Build history of the part. All positions in model axes, mm. A direction names the side the tool comes from. Round coordinates to 2 decimals unless told otherwise and drop trailing zeros. Write each loop counter-clockwise with the first axis right and the second up, starting at its lowest first coordinate (ties: lowest second). Pieces come first, ordered by that corner, then holes.
1) Which spindle directions (+Z, -Z, +X, -X, +Y, -Y) get a long thin tool onto all of the face, cutting with end or side? Do faces 4 (the flat face through (15.76, -5.42, -0.91)), 5 (the flat face through (14, -11, -12)), 6 (the flat face through (16.257, -5.423, -9.902)). Say none if no direction does.
2) Flat gauge pins, fed straight in: pin 1 (4 mm diameter, centred on y = -5.5, z = -5, fed in from -X); pin 2 (6 mm diameter, centred on x = 1.5, y = -4, fed in from -Z); pin 3 (1 mm diameter, centred on y = -2, z = -7, fed in from +X); pin 4 (14 mm diameter, centred on x = -4.5, z = -2, fed in from -Y). Where does each tip first touch, or does it go through?
3) Saw through at D-D (x = 19.5). Write the cut outline in (y, z).
4) Wall check: probe 1 along Y at (x, z) = (9, 7.75); probe 2 along X at (y, z) = (0.35, 0); probe 3 along Z at (x, y) = (14, -1). Give the ranges that are in metal, low to high.
5) Saw through at A-A (y = -7). Write the cut outline in (x, z).
6) Saw through at C-C (z = -8). Write the cut outline in (x, y).
7) Saw through at B-B (x = -6). Write the cut outline in (y, z).
8) Pull direction X, two halves, no side cores. Call faces 1 (the flat face through (18.617, -5.423, -6.194)), 2 (the flat face through (19, -11, -6)), 3 (the cylindrical face through (11.68, -5.42, -10.98)): +X half, -X half, draft (parallel to the pull), parting line (faces both ways), or undercut.
from build123d import *

# Parameters (mm, degrees)
SKETCH1_R           = 14
BOSS_EXTRUDE1_DEPTH = 1
BOSS_EXTRUDE2_DEPTH = 11
BOSS_EXTRUDE3_DEPTH = 11
SKETCH4_R           = 10
CUT_EXTRUDE1_DEPTH  = 11


with BuildPart() as part:
    # Sketch1 → Boss-Extrude1 (new body)
    with BuildSketch(Plane(origin=(0, 0, 0), x_dir=(1, 0, 0), z_dir=(0, 1, 0))):
        Circle(SKETCH1_R)
        with BuildLine():
            Line((14.805399496, 14), (0, 14))
            ThreePointArc((0, 14), (9.899494937, 9.899494937), (14, 0))
            ThreePointArc((14, 0), (13.900075645, -1.66969969), (13.601728992, -3.31556457))
            Line((13.601728992, -3.31556457), (22.770248109, 10.778060096))
            Line((22.770248109, 10.778060096), (14.805399496, 14))
        make_face()
    extrude(amount=BOSS_EXTRUDE1_DEPTH)

    # Sketch2 → Boss-Extrude2 (add)
    with BuildSketch(Plane(origin=(0, 0, 0), x_dir=(-1, 0, 0), z_dir=(0, -1, 0))):
        Polygon((-22.770248109, 10.778060096), (-21.843223298, 11.153060096), (-15.299518751, 1.094236567), (-16.226543561, 0.719236567), align=None)
    extrude(amount=BOSS_EXTRUDE2_DEPTH)

    # Sketch3 → Boss-Extrude3 (add)
    with BuildSketch(Plane(origin=(0, 0, 0), x_dir=(-1, 0, 0), z_dir=(0, -1, 0))):
        with BuildLine():
            Line((-18.06544552, 12.681246451), (-14.398150781, 7.043970142))
            ThreePointArc((-14.398150781, 7.043970142), (-11.63382994, 11.026253317), (-7.805399496, 14))
            Line((-7.805399496, 14), (-14.805399496, 14))
            Line((-14.805399496, 14), (-18.06544552, 12.681246451))
        make_face()
    extrude(amount=BOSS_EXTRUDE3_DEPTH)

    # Sketch4 → Cut-Extrude1 (cut)
    with BuildSketch(Plane.XZ):
        with Locations(Location((0, 0, 0), (0, 0, 270))):
            Circle(SKETCH4_R)
    extrude(amount=-CUT_EXTRUDE1_DEPTH, mode=Mode.SUBTRACT)


solid = part.part
Evaluation:
1. face 4: +Z, -X, -Y
1. face 5: +Z, -Z, +X, -X, -Y
1. face 6: -Y
2. pin 1: stops at x = 16.54
2. pin 2: passes through
2. pin 3: stops at x = 20.64
2. pin 4: stops at y = 0
3. outline: (-11, -7.55) - (0, -7.55) - (0, -12.1) - (1, -12.1) - (1, -5.75) - (-11, -5.75) - close
4. probe 1: y = 0 to 1
4. probe 2: x = -14 to -10, 10 to 15.76
4. probe 3: z = -14 to -7.81
5. outline: (7.81, -14) - (14.81, -14) - (18.07, -12.68) - (14.4, -7.04) arc R16.03 cw to start; (15.3, -1.09) - (21.84, -11.15) - (22.77, -10.78) - (16.23, -0.72) - close
6. outline: (-11.49, 0) - (-6, 0) - (-6, 1) - (-11.49, 1) - close; (6, 0) - (13.89, 0) - (13.89, -11) - (15.02, -11) - (15.02, 0) - (19.79, 0) - (19.79, -11) - (20.96, -11) - (20.96, 1) - (6, 1) - close
7. outline: (0, -12.65) - (1, -12.65) - (1, -8) - (0, -8) - close; (0, 8) - (1, 8) - (1, 12.65) - (0, 12.65) - close
8. face 1: undercut
8. face 2: draft
8. face 3: -X half
